Input: part model. Units: mm. Frame: model coordinates. A direction names the side the tool comes from. Coordinates: 2 decimals unless noted, no trailing zeros. Loops run counter-clockwise (first coordinate to the right, second up) from the corner with the lowest first, then second, coordinate; pieces in that order, holes last. Notation, with made-up numbers: (-16.5, 72) - (9.5, 72) arc R34 cw to (9.5, 104) - close; hole circle Ø9 at (19.5, 83). An arc over 180 degrees is marked (long way). Use one line per item in the form item = value.
from build123d import *

# Parameters (mm, degrees)
SKETCH1_W           = 10.16
SKETCH1_H           = 20.32
SKETCH1_R           = 2.50063
BOSS_EXTRUDE1_DEPTH = 2.54
SKETCH2_W           = 10.16
SKETCH2_H           = 2.564193751
BOSS_EXTRUDE2_DEPTH = 19.05
SKETCH3_R           = 3.175
CUT_EXTRUDE1_DEPTH  = 2.564193751


with BuildPart() as part:
    # Sketch1 → Boss-Extrude1 (new body)
    with BuildSketch(Plane(origin=(0, 0, 0), x_dir=(1, 0, 0), z_dir=(0, 1, 0))):
        Rectangle(SKETCH1_W, SKETCH1_H)
        with Locations(Location((0, 6.35, 0), (0, 0, 270))):
            Circle(SKETCH1_R, mode=Mode.SUBTRACT)
        with Locations(Location((0, -3.81, 0), (0, 0, 270))):
            Circle(SKETCH1_R, mode=Mode.SUBTRACT)
    extrude(amount=BOSS_EXTRUDE1_DEPTH)

    # Sketch2 → Boss-Extrude2 (add)
    with BuildSketch(Plane(origin=(0, 2.54, 0), x_dir=(1, 0, 0), z_dir=(0, 1, 0))):
        with Locations((0, -8.877903125)):
            Rectangle(SKETCH2_W, SKETCH2_H)
    extrude(amount=BOSS_EXTRUDE2_DEPTH)

    # Sketch3 → Cut-Extrude1 (cut)
    with BuildSketch(Plane.XY.offset(10.16)):
        with Locations((0, 13.589)):
            Circle(SKETCH3_R)
    extrude(amount=-CUT_EXTRUDE1_DEPTH, mode=Mode.SUBTRACT)


solid = part.part
Q1. Set-up query: faces 1 (the flat face through (0, 2.54, -1)), 2 (the flat face through (0, 1, -10.16)). Return all of +Z, -Z, +X, -X, +Y, -Y with unobstructed straight access to the full face (end or side cutting, diameter ignored); none if empty.
Check values:
face_1 = -Z, +X, -X, +Y
face_2 = -Z, +X, -X, +Y, -Y
Q2. Cut plane C-C, the plane z = -8. Return loops of the section in (x, y), then the cut area to 3 significant figures.
Check values:
outline = (-5.08, 0) - (-1.88, 0) - (-1.88, 2.54) - (-5.08, 2.54) - close; (1.88, 0) - (5.08, 0) - (5.08, 2.54) - (1.88, 2.54) - close
area = 16.3 mm²
Q3. First-contact query: P1, Ø5.5, axis at x = 0, y = 13.589, coming from the -Z side; P2, Ø5, axis at x = -3, y = 19, coming from the -Z side; P3, Ø3, axis at x = -2, z = 3, coming from the +Y side. Flat tips, straight axial feed; report the tip coordinate or a pass-through.
Check values:
P1 = through
P2 = 7.6
P3 = 2.54
Q4. Cut plane A-A, the plane z = 3.81. Return loops of the section in (x, y).
Check values:
outline = (-5.08, 0) - (-2.5, 0) - (-2.5, 2.54) - (-5.08, 2.54) - close; (2.5, 0) - (5.08, 0) - (5.08, 2.54) - (2.5, 2.54) - close
Q5. Cut plane D-D, the plane x = 1.5. Return loops of the section in (y, z).
Check values:
outline = (0, -10.16) - (2.54, -10.16) - (2.54, -8.35) - (0, -8.35) - close; (0, -4.35) - (2.54, -4.35) - (2.54, 1.81) - (0, 1.81) - close; (0, 5.81) - (2.54, 5.81) - (2.54, 7.6) - (10.79, 7.6) - (10.79, 10.16) - (0, 10.16) - close; (16.39, 7.6) - (21.59, 7.6) - (21.59, 10.16) - (16.39, 10.16) - close
Q6. Cut plane B-B, the plane x = 0. Return loops of the section in (y, z).
Check values:
outline = (0, -10.16) - (2.54, -10.16) - (2.54, -8.85) - (0, -8.85) - close; (0, -3.85) - (2.54, -3.85) - (2.54, 1.31) - (0, 1.31) - close; (0, 6.31) - (2.54, 6.31) - (2.54, 7.6) - (10.41, 7.6) - (10.41, 10.16) - (0, 10.16) - close; (16.76, 7.6) - (21.59, 7.6) - (21.59, 10.16) - (16.76, 10.16) - close
Q7. Pull-direction query (Z, two-part tool) for faces 3 (the flat face through (0, 10, 7.596)), 4 (the flat face through (5.08, 6, 8)), 5 (the cylindrical face through (-1.522, 1.252, 1.826)); classes: pulls with the +Z half, pulls with the -Z half, needs draft (parallel to the pull), parting line crosses it, or undercut.
Check values:
face_3 = pulls with the -Z half
face_4 = needs draft
face_5 = undercut
Q8. Ray query, line 1 along Y through (x, z) = (0, 9.45); line 2 along Z through (x, y) = (-1, 1); line 3 along Z through (x, y) = (4.25, 12). Return the intervals inside material, ascending. Write a range as [from, to].
Check values:
line_1 = [0, 10.41], [16.76, 21.59]
line_2 = [-10.16, -8.64], [-4.06, 1.52], [6.1, 10.16]
line_3 = [7.6, 10.16]
